Design review of the part built by this model. Coordinates are the model's own, in mm. A direction names the side the tool comes from. Round coordinates to 2 decimals unless told otherwise and drop trailing zeros. Write each loop counter-clockwise with the first axis right and the second up, starting at its lowest first coordinate (ties: lowest second). Pieces come first, ordered by that corner, then holes. Notation, with made-up numbers: (10, -38) -> (59, -38) arc R11 ccw to (59, -34) -> close; hole circle Ø6 at (51, 4). An arc over 180 degrees is marked (long way). One line per question, with ' | ' between items. Start each with the question number.
1) Mouldability with a two-part tool opening along X and no side actions: class faces 1 (the flat face through (3.5, 2, 2)), 2 (the flat face through (3.2, 2.3, 5)), 3 (the flat face through (-0.5, 2, 2)), 4 (the flat face through (0, 2, 2)) as +X half, -X half, draft (parallel to the pull), parting line (faces both ways), or undercut.
2) For probe 1 along Y at (x, z) = (0.3, 3.5); probe 2 along X at (y, z) = (0.7, 3.55); probe 3 along Z at (x, y) = (1.5, 4.75), list the stretches that pass through material, from the lowest coordinate up.
3) Consider section C-C (x = 1.5). Give the boundary of the cut face in (y, z).
4) Consider section A-A (y = 1.9). Give the boundary of the cut face in (x, z).
5) Consider section D-D (z = 3.65). Give the boundary of the cut face in (x, y).
6) Consider section B-B (x = 2.45). Give the boundary of the cut face in (y, z).
7) For faces 5 (the cylindrical face through (1.903, 4.754, 1.868)), 6 (the flat face through (0.6, 5, 2.5)), 7 (the flat face through (1, 0, 2)), list the 3-axis set-ups (+Z, -Z, +X, -X, +Y, -Y) from which the entire face can be reached by the end or side of a thin tool; tool diameter is ignored.
```python
from build123d import *

# Parameters (mm, degrees)
SKETCH1_W           = 4
SKETCH1_H           = 5.5
SKETCH1_W_2         = 3
SKETCH1_H_2         = 4.5
EXTRUDE_THIN1_DEPTH = 5
CUT_EXTRUDE1_REACH  = 7.5
SKETCH2_R           = 0.75


with BuildPart() as part:
    # Sketch1 → Extrude-Thin1 (new body)
    with BuildSketch(Plane.XY):
        with Locations((1.5, 2.25)):
            Rectangle(SKETCH1_W, SKETCH1_H)
        with Locations((1.5, 2.25)):
            Rectangle(SKETCH1_W_2, SKETCH1_H_2, mode=Mode.SUBTRACT)
    extrude(amount=EXTRUDE_THIN1_DEPTH)

    # Sketch2 → Cut-Extrude1 (cut, up to next)
    with BuildSketch(Plane(origin=(0, 5, 0), x_dir=(1, 0, 0), z_dir=(0, 1, 0)), mode=Mode.PRIVATE) as cut_extrude1_sk1:
        with Locations((1.5, -2.5)):
            Circle(SKETCH2_R)
    cut_extrude1_tool1 = extrude(cut_extrude1_sk1.sketch, amount=-CUT_EXTRUDE1_REACH, mode=Mode.PRIVATE) & part.part
    add(cut_extrude1_tool1.solids().sort_by_distance((1.5, 5, 2.5))[0], mode=Mode.SUBTRACT)


solid = part.part
```
From the geometry:
1) face 1: +X half | face 2: draft | face 3: -X half | face 4: undercut
2) probe 1: y = -0.5 to 0, 4.5 to 5 | probe 2: x = -0.5 to 0, 3 to 3.5 | probe 3: z = 0 to 1.75, 3.25 to 5
3) outline: (-0.5, 0) -> (0, 0) -> (0, 5) -> (-0.5, 5) -> close; (4.5, 0) -> (5, 0) -> (5, 1.75) -> (4.5, 1.75) -> close; (4.5, 3.25) -> (5, 3.25) -> (5, 5) -> (4.5, 5) -> close
4) outline: (-0.5, 0) -> (0, 0) -> (0, 5) -> (-0.5, 5) -> close; (3, 0) -> (3.5, 0) -> (3.5, 5) -> (3, 5) -> close
5) outline: (-0.5, -0.5) -> (3.5, -0.5) -> (3.5, 5) -> (-0.5, 5) -> close; hole (0, 0) -> (3, 0) -> (3, 4.5) -> (0, 4.5) -> close
6) outline: (-0.5, 0) -> (0, 0) -> (0, 5) -> (-0.5, 5) -> close; (4.5, 0) -> (5, 0) -> (5, 5) -> (4.5, 5) -> close
7) face 5: +Y | face 6: +Z, -Z, +X, -X, +Y | face 7: +Z, -Z
